Model file for the job. Use its own axes, mm. A direction names the side the tool comes from. Coordinates: 2 decimals unless noted, no trailing zeros. Order: outer loops, then holes, each group sorted by start corner. A loop starts at its lowest first (then second) coordinate and runs counter-clockwise, first axis right, second up. Notation, with made-up numbers: (-20.5, 55) -> (7.5, 55) arc R22 cw to (7.5, 67) -> close; hole circle Ø2 at (71, -17). An arc over 180 degrees is marked (long way). Return JSON: item names as keys, results as strings. Group by question number.
1) Probe line 1 (X direction, y = 7, z = -1021); line 2 (Y direction, x = 11.5, z = -249.5); line 3 (Y direction, x = -4.5, z = -211). List the from-to ranges inside material, lowest first.
2) Cut at B-B (y = 19.5). Write the cut outline in (x, z).
3) Flat gauge pins, fed straight in: pin 1 (4 mm diameter, centred on x = -7, z = -981.5, fed in from +Y); pin 2 (12 mm diameter, centred on x = -13.5, z = -1186, fed in from +Y); pin 3 (1.5 mm diameter, centred on x = -14.5, z = -1268, fed in from +Y). Where does each tip first touch, or does it go through?
4) Which spindle directions (+Z, -Z, +X, -X, +Y, -Y) get a long thin tool onto all of the face, cutting with end or side? Do faces 1 (the flat face through (28.323, 19.728, -713.765)), 2 (the flat face through (-27.341, 19.465, -713.765)). Say none if no direction does.
5) Cut at A-A (z = -793.5). Write the cut outline in (x, y).
6) Pull direction Y, two halves, no side cores. Call faces 3 (the flat face through (-2.6, 0.7, -1447.8)), 4 (the flat face through (27.22, 19.91, -713.77)), 5 (the flat face through (-28.204, 20.171, -713.765)): +Y half, -Y half, draft (parallel to the pull), parting line (faces both ways), or undercut.
from build123d import *

# Parameters (mm, degrees)
BASE_FLANGE1_DEPTH = 1447.8


# Sheet-metal steps are written as plain solids
with BuildPart() as part:
    # Sketch1 → Base-Flange1 (new body)
    with BuildSketch(Plane.XY):
        with BuildLine():
            Line((-24.017856008, 35.793752438), (-32.508689678, 4.105529785))
            ThreePointArc((-32.508689678, 4.105529785), (-32.247725893, 2.625530619), (-30.946236469, 1.87411535))
            Line((-30.946236469, 1.87411535), (-9.602333754, 0.006765827))
            ThreePointArc((-9.602333754, 0.006765827), (-9.524926114, 0.001692262), (-9.447370844, 0))
            Line((-9.447370844, 0), (9.447370844, 0))
            ThreePointArc((9.447370844, 0), (9.524926114, 0.001692262), (9.602333754, 0.006765827))
            Line((9.602333754, 0.006765827), (30.946236469, 1.87411535))
            ThreePointArc((30.946236469, 1.87411535), (32.247725893, 2.625530619), (32.508689678, 4.105529785))
            Line((32.508689678, 4.105529785), (24.017856008, 35.793752438))
            Line((24.017856008, 35.793752438), (23.036475369, 35.530792289))
            Line((23.036475369, 35.530792289), (31.527309038, 3.842569635))
            ThreePointArc((31.527309038, 3.842569635), (31.415467416, 3.208284278), (30.857686234, 2.886249163))
            Line((30.857686234, 2.886249163), (9.513783519, 1.01889964))
            ThreePointArc((9.513783519, 1.01889964), (9.480608817, 1.016725255), (9.447370844, 1.016))
            Line((9.447370844, 1.016), (-9.447370844, 1.016))
            ThreePointArc((-9.447370844, 1.016), (-9.480608817, 1.016725255), (-9.513783519, 1.01889964))
            Line((-9.513783519, 1.01889964), (-30.857686234, 2.886249163))
            ThreePointArc((-30.857686234, 2.886249163), (-31.415467416, 3.208284278), (-31.527309038, 3.842569635))
            Line((-31.527309038, 3.842569635), (-23.036475369, 35.530792289))
            Line((-23.036475369, 35.530792289), (-24.017856008, 35.793752438))
        make_face()
    extrude(amount=-BASE_FLANGE1_DEPTH)


solid = part.part
Answers below:
{
 "1": {"line 1": "x = -31.73 to -30.68, 30.68 to 31.73", "line 2": "y = 0.17 to 1.19", "line 3": "y = 0 to 1.02"},
 "2": {"outline": "(-28.38, -1447.8) -> (-27.33, -1447.8) -> (-27.33, 0) -> (-28.38, 0) -> close; (27.33, -1447.8) -> (28.38, -1447.8) -> (28.38, 0) -> (27.33, 0) -> close"},
 "3": {"pin 1": "stops at y = 1.02", "pin 2": "stops at y = 1.89", "pin 3": "stops at y = 1.52"},
 "4": {"face 1": "+Z, -Z, +X, +Y", "face 2": "+Z, -Z"},
 "5": {"outline": "(-32.51, 4.11) arc R1.78 ccw to (-30.95, 1.87) -> (-9.6, 0.01) arc R1.78 ccw to (-9.45, 0) -> (9.45, 0) arc R1.78 ccw to (9.6, 0.01) -> (30.95, 1.87) arc R1.78 ccw to (32.51, 4.11) -> (24.02, 35.79) -> (23.04, 35.53) -> (31.53, 3.84) arc R0.76 cw to (30.86, 2.89) -> (9.51, 1.02) arc R0.76 cw to (9.45, 1.02) -> (-9.45, 1.02) arc R0.76 cw to (-9.51, 1.02) -> (-30.86, 2.89) arc R0.76 cw to (-31.53, 3.84) -> (-23.04, 35.53) -> (-24.02, 35.79) -> close"},
 "6": {"face 3": "draft", "face 4": "undercut", "face 5": "+Y half"}
}
